from build123d import *

# Parameters (mm, degrees)
SKETCH1_R           = 3.175
BOSS_EXTRUDE1_DEPTH = 406.4
SKETCH2_W           = 25.4
SKETCH2_H           = 12.7
CUT_EXTRUDE1_DEPTH  = 11.922
LPATTERN1_COUNT     = 8
LPATTERN1_PITCH     = 50.8
SKETCH3_R           = 4.7625
CUT_EXTRUDE2_DEPTH  = 3.286


with BuildPart() as part:
    # Sketch1 → Boss-Extrude1 (new body)
    with BuildSketch(Plane.XY):
        with BuildLine():
            Line((5.461, 0), (5.461, -38.1))
            Line((5.461, -38.1), (3.175, -38.1))
            Line((3.175, -38.1), (3.175, -4.443185344))
            ThreePointArc((3.175, -4.443185344), (-4.855985791, 2.498384078), (5.461, 0))
        make_face()
        Circle(SKETCH1_R, mode=Mode.SUBTRACT)
    extrude(amount=BOSS_EXTRUDE1_DEPTH)

    # Sketch2 → Cut-Extrude1 (cut, through all)
    with BuildSketch(Plane(origin=(5.461, 0, 0), x_dir=(0, 0, -1), z_dir=(1, 0, 0))):
        with Locations((-393.7, -0.889)):
            Rectangle(SKETCH2_W, SKETCH2_H)
    cut_extrude1 = extrude(amount=-CUT_EXTRUDE1_DEPTH, mode=Mode.SUBTRACT)

    # LPattern1: Cut-Extrude1 ×8
    with Locations(*[(0, 0, -i * LPATTERN1_PITCH) for i in range(1, LPATTERN1_COUNT)]):
        add(cut_extrude1, mode=Mode.SUBTRACT)

    # Sketch3 → Cut-Extrude2 (cut, through all)
    with BuildSketch(Plane.ZY.offset(-3.175)):
        with Locations((25.4, -22.6695)):
            Circle(SKETCH3_R)
        with Locations((203.2, -22.6695)):
            Circle(SKETCH3_R)
        with Locations((381, -22.6695)):
            Circle(SKETCH3_R)
    extrude(amount=-CUT_EXTRUDE2_DEPTH, mode=Mode.SUBTRACT)


solid = part.part
CAD build for the part. Positions are in the model's coordinates, mm. A direction names the side the tool comes from. Round coordinates to 2 decimals unless told otherwise and drop trailing zeros. Order: outer loops, then holes, each group sorted by start corner. A loop starts at its lowest first (then second) coordinate and runs counter-clockwise, first axis right, second up. Notation, with made-up numbers: (81, -11) - (138, -11) arc R12 ccw to (138, 10) - close; hole circle Ø10 at (12.25, 83). An arc over 180 degrees is marked (long way). Return JSON: item names as keys, results as strings.
(1) Pin check, flat tips, straight feed: pin 1 Ø3.5 at (x, y) = (0.5, 2) entering from +Z; pin 2 Ø0.7 at (x, z) = (5, 389) entering from +Y; pin 3 Ø5 at (y, z) = (-11.5, 98) entering from -X (3 decimals). Stop position of each tip, or through.
Answer key:
{"pin 1": "stops at z = 381", "pin 2": "stops at y = -7.24", "pin 3": "stops at x = 3.175"}
(2) Wall check: probe 1 along Y at (x, z) = (0, 311.75) (3 decimals); probe 2 along Y at (x, z) = (4.5, 130); probe 3 along X at (y, z) = (-34.5, 126) (3 decimals). Give the ranges that are in metal, low to high. Write a range as from..to.
Answer key:
{"probe 1": "y = -5.461..-3.175, 3.175..5.461", "probe 2": "y = -38.1..-7.24", "probe 3": "x = 3.175..5.461"}
(3) Cut at B-B (z = 340.5). Give the cut face in (x, y) (3 decimals), then the cut area to 3 significant figures.
Answer key:
{"outline": "(3.175, -38.1) - (5.461, -38.1) - (5.461, -7.239) - (3.175, -7.239) - close", "area": "70.5 mm^2"}
(4) Tool access for faces 4 (the face through (3, -2, 50.8)), 5 (the face through (-0.69, -3.1, 368.12)): list every direction of +Z, -Z, +X, -X, +Y, -Y with a clear straight run to the whole face (end or side of a thin tool).
Answer key:
{"face 4": "+X, -X, +Y", "face 5": "+Z, -Z"}
(5) Pull direction X, two halves, no side cores. Call faces 1 (the face through (3, -2, 203.2)), 2 (the face through (-0.69, -3.1, 114.12)), 3 (the face through (5.461, -15, 200)): +X half, -X half, draft (parallel to the pull), parting line (faces both ways), or undercut.
Answer key:
{"face 1": "draft", "face 2": "undercut", "face 3": "+X half"}
(6) Cut at A-A (x = 0). State how many separate pieces and enclosed holes the cut face has, then the cut area to 3 significant figures.
Answer key:
{"separate pieces": "16", "enclosed holes": "0", "area": "929 mm^2"}
